Geometry: final body of the model. Coordinates: model frame, mm. Face numbers are marked on the shaded views. A direction names the side the tool comes from. Give positions to 0.01 mm unless a question says otherwise; leave off trailing zeros. Write each loop counter-clockwise with the first axis right and the second up, starting at its lowest first coordinate (ties: lowest second). Pieces come first, ordered by that corner, then holes.
from build123d import *

# Parameters (mm, degrees)
CUT_EXTRUDE1_DEPTH = 2
CHAMFER1_SIZE      = 0.4
CHAMFER2_SIZE      = 0.1


with BuildPart() as part:
    # Sketch2 → Revolve1 (revolve)
    with BuildSketch(Plane(origin=(0, 0, 0), x_dir=(0, 0, -1), z_dir=(1, 0, 0))):
        Polygon((0, 2.5), (-2, 2.5), (-2, 1.5), (-5, 1.5), (-5, 0), (0, 0), align=None)
    revolve(axis=Axis((0, 0, 5), (0, 0, -1)))

    # Sketch3 → Cut-Extrude1 (cut)
    with BuildSketch(Plane(origin=(0, 0, 0), x_dir=(-1, 0, 0), z_dir=(0, 0, -1))):
        Polygon((1.168445951, -0.498063644), (1.015558744, 0.762872054), (-0.152887207, 1.260935698), (-1.168445951, 0.498063644), (-1.015558744, -0.762872054), (0.152887207, -1.260935698), align=None)
    extrude(amount=-CUT_EXTRUDE1_DEPTH, mode=Mode.SUBTRACT)

    # Chamfer1
    chamfer1_edges = [part.edges().sort_by_distance(p)[0] for p in [
        (0, -1.5, 5),
        (0, -2.5, 0),
    ]]
    chamfer(chamfer1_edges, length=CHAMFER1_SIZE)

    # Chamfer2
    chamfer2_edges = [part.edges().sort_by_distance(p)[0] for p in [
        (-0.660666579, -0.879499671, 0),
        (-1.092002347, 0.132404205, 0),
        (-0.431335769, 1.011903876, 0),
        (0.660666579, 0.879499671, 0),
        (1.092002347, -0.132404205, 0),
        (0.431335769, -1.011903876, 0),
    ]]
    chamfer(chamfer2_edges, length=CHAMFER2_SIZE)


solid = part.part
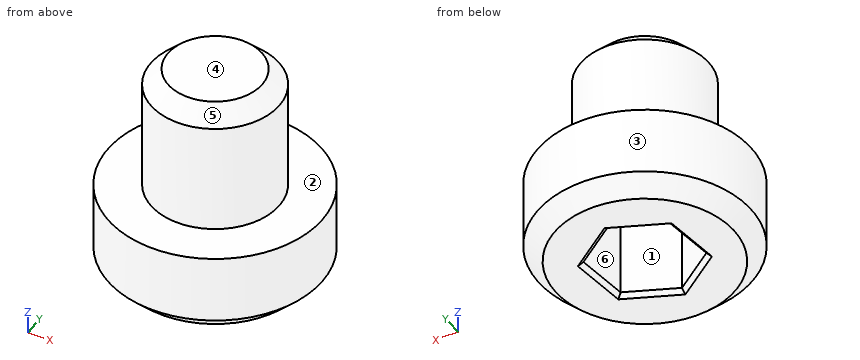
Q1. Ray query, line 1 along Z through (x, y) = (1.05, 1.2); line 2 along Z through (x, y) = (-0.9, 0.4); line 3 along X through (y, z) = (0, 3.25). Return the intervals inside material, ascending.
Filled sheet:
line 1: z = 0 to 2
line 2: z = 2 to 5
line 3: x = -1.5 to 1.5
Q2. Section D-D on x = 0. Output: boundary loops of the cut face in (y, z), plus the area to 3 significant figures.
Filled sheet:
outline: (-2.5, 0.4) - (-2.1, 0) - (-1.3, 0) - (-1.2, 0.1) - (-1.2, 2) - (1.2, 2) - (1.2, 0.1) - (1.3, 0) - (2.1, 0) - (2.5, 0.4) - (2.5, 2) - (1.5, 2) - (1.5, 4.6) - (1.1, 5) - (-1.1, 5) - (-1.5, 4.6) - (-1.5, 2) - (-2.5, 2) - close
area: 13.9 mm2
Q3. Access query for the marked faces 1, 2 and 3. Directions: +Z, -Z, +X, -X, +Y, -Y. A direction counts if a zero-diameter tool reaches every point of the face in a straight line with its end or side. Return the directions, or none.
Filled sheet:
face 1: -Z
face 2: +Z
face 3: +Z, -Z
Q4. Section A-A on z = 1.4. Output: boundary loops of the cut face in (x, y), plus the area to 3 significant figures.
Filled sheet:
outline: circle Ø5 at (0, 0); hole (-1.17, -0.5) - (-0.15, -1.26) - (1.02, -0.76) - (1.17, 0.5) - (0.15, 1.26) - (-1.02, 0.76) - close
area: 15.4 mm2
Q5. Pin query (flat end, axial travel): P1, Ø1.2, axis at x = 0, y = 0, coming from the -Z side. Return the tip coordinate at first contact, or that it passes through.
Filled sheet:
P1: stops at z = 2
Q6. Section B-B on y = 0. Output: boundary loops of the cut face in (x, z).
Filled sheet:
outline: (-2.5, 0.4) - (-2.1, 0) - (-1.21, 0) - (-1.11, 0.1) - (-1.11, 2) - (1.11, 2) - (1.11, 0.1) - (1.21, 0) - (2.1, 0) - (2.5, 0.4) - (2.5, 2) - (1.5, 2) - (1.5, 4.6) - (1.1, 5) - (-1.1, 5) - (-1.5, 4.6) - (-1.5, 2) - (-2.5, 2) - close
Q7. Pull-direction query (Y, two-part tool) for the marked faces 4, 5 and 6; classes: released by +Y, released by -Y, zero draft, split by the parting line, or undercut.
Filled sheet:
face 4: zero draft
face 5: split by the parting line
face 6: undercut
Q8. Section C-C on z = 4.3. Output: boundary loops of the cut face in (x, y).
Filled sheet:
outline: circle Ø3 at (0, 0)
